```python
from build123d import *
from OCP.BRepFilletAPI import BRepFilletAPI_MakeChamfer

# Parameters (mm, degrees)
SKETCH1_R            = 4.999999999999999
SKETCH1_R_2          = 2.5
BOSS_EXTRUDE1_DEPTH  = 15.8
SKETCH2_R            = 3.75
CUT_EXTRUDE1_DEPTH   = 13
CUT_EXTRUDE2_DEPTH   = 19.135324645563973
BOSS_EXTRUDE3_DEPTH  = 1
BOSS_EXTRUDE4_DEPTH  = 1
SKETCH13_R           = 5
BOSS_EXTRUDE7_DEPTH  = 10
CUT_EXTRUDE3_START   = -4
CUT_EXTRUDE3_DEPTH   = 4
CUT_EXTRUDE4_DEPTH   = 1
BOSS_EXTRUDE9_DEPTH  = 3
CUT_EXTRUDE6_DEPTH   = 7
BOSS_EXTRUDE10_DEPTH = 3
BOSS_EXTRUDE11_DEPTH = 2
CUT_EXTRUDE7_DEPTH   = 0.25
BOSS_EXTRUDE12_DEPTH = 1
SKETCH23_W           = 18.9749371855331
SKETCH23_H           = 13
BOSS_EXTRUDE13_DEPTH = 1
SKETCH24_W           = 23.799999999999997
SKETCH24_H           = 13
BOSS_EXTRUDE14_DEPTH = 1
BOSS_EXTRUDE15_DEPTH = 1
SKETCH26_W           = 11.45
SKETCH26_H           = 6.999999999999998
SKETCH26_W_2         = 10.45
SKETCH26_H_2         = 5.999999999999998
CUT_EXTRUDE8_DEPTH   = 34.46489573009899
CUT_EXTRUDE10_DEPTH  = 0.7
CHAMFER4_SIZE        = 0.8
CHAMFER4_SIZE2       = 2.1979819355637176


with BuildPart() as part:
    # Sketch1 → Boss-Extrude1 (new body)
    # profile 1 of 2: a face of its own
    with BuildSketch(Plane(origin=(0, 0, 0), x_dir=(1, 0, 0), z_dir=(0, 1, 0))):
        with BuildLine():
            Line((-0.5, 7), (-0.5, 4.9749371855331))
            ThreePointArc((-0.5000000000000004, 4.974937185533099), (3.1e-16, 4.999999999999999), (0.49999999999999994, 4.974937185533099))
            Line((0.5, 4.9749371855331), (0.5, 7))
            Line((0.5, 7), (-0.5, 7))
        make_face()
    # profile 2 of 2: a face of its own
    with BuildSketch(Plane(origin=(0, 0, 0), x_dir=(1, 0, 0), z_dir=(0, 1, 0))):
        Circle(SKETCH1_R)
        with Locations(Location((0, 0, 0), (0, 0, 270))):
            Circle(SKETCH1_R_2, mode=Mode.SUBTRACT)
    extrude(amount=BOSS_EXTRUDE1_DEPTH)

    # Sketch2 → Cut-Extrude1 (cut)
    with BuildSketch(Plane(origin=(0, 15.8, 0), x_dir=(1, 0, 0), z_dir=(0, 1, 0))):
        with Locations(Location((0, 0, 0), (0, 0, 270))):
            Circle(SKETCH2_R)
    extrude(amount=-CUT_EXTRUDE1_DEPTH, mode=Mode.SUBTRACT)

    # Sketch4 → Cut-Extrude2 (cut, through all)
    with BuildSketch(Plane(origin=(0.5, 0, 0), x_dir=(0, 0, -1), z_dir=(1, 0, 0))):
        Polygon((7, 0), (4.9749371855331, 0), (4.9749371855331, 2.5000000000000004), (7, 2.5), align=None)
    extrude(amount=-CUT_EXTRUDE2_DEPTH, mode=Mode.SUBTRACT)

    # Sketch10 → Boss-Extrude3 (add)
    with BuildSketch(Plane(origin=(0.5, 0, 0), x_dir=(0, 0, -1), z_dir=(1, 0, 0))):
        Polygon((4.9749371855331, 15.8), (9.974937185533099, 15.8), (9.974937185533099, 9.8), (4.974937185533101, 9.8), align=None)
    extrude(amount=-BOSS_EXTRUDE3_DEPTH)

    # Sketch12 → Boss-Extrude4 (add)
    with BuildSketch(Plane(origin=(0, 15.8, 0), x_dir=(1, 0, 0), z_dir=(0, 1, 0))):
        with BuildLine():
            Line((-3.75, -3.307189138830739), (-3.75, 3.307189138830739))
            ThreePointArc((-3.75, 3.307189138830739), (-5.000000000000001, -6.1e-16), (-3.75, -3.307189138830739))
        make_face()
    extrude(amount=BOSS_EXTRUDE4_DEPTH)

    # Sketch13 → Boss-Extrude7 (add)
    with BuildSketch(Plane.XZ.offset(-9.8)):
        Polygon((-8, 8), (14.799999999999997, 8), (14.8, -9.974937185533099), (-7.999999999999998, -9.974937185533099), align=None)
        with Locations(Location((0, 0, 0), (0, 0, 221.409622109))):
            Circle(SKETCH13_R, mode=Mode.SUBTRACT)
    extrude(amount=-BOSS_EXTRUDE7_DEPTH)

    # Sketch14 → Cut-Extrude3 (cut)
    with BuildSketch(Plane(origin=(0, 19.8, 0), x_dir=(1, 0, 0), z_dir=(0, 1, 0)).offset(CUT_EXTRUDE3_START)):
        Polygon((-4.400000000000001, 5.7), (10.299999999999999, 5.7), (12.899999999999999, 5.7), (12.899999999999999, -7.249999999999999), (10.3, -7.249999999999999), (-4.400000000000001, -7.249999999999999), align=None)
    extrude(amount=CUT_EXTRUDE3_DEPTH, mode=Mode.SUBTRACT)

    # Sketch15 → Cut-Extrude4 (cut)
    with BuildSketch(Plane(origin=(0, 19.8, 0), x_dir=(1, 0, 0), z_dir=(0, 1, 0))):
        Polygon((-7.499999999999998, 9.474937185533099), (-7.5, -7.5), (14.299999999999997, -7.5), (14.3, 9.474937185533099), align=None)
    extrude(amount=-CUT_EXTRUDE4_DEPTH, mode=Mode.SUBTRACT)

    # Sketch17 → Boss-Extrude9 (add)
    with BuildSketch(Plane.XZ.offset(-9.8)):
        Polygon((14.8, -5.974937185533098), (4.3, -5.974937185533099), (4.3, 8), (14.8, 8), align=None)
    extrude(amount=BOSS_EXTRUDE9_DEPTH)

    # Sketch16 → Cut-Extrude6 (cut)
    with BuildSketch(Plane(origin=(0, 15.8, 0), x_dir=(1, 0, 0), z_dir=(0, 1, 0))):
        Polygon((12.899999999999999, 5.7), (4.999999999999999, 5.699999999999999), (5.000000000000001, -7.249999999999999), (12.9, -7.249999999999999), align=None)
    extrude(amount=-CUT_EXTRUDE6_DEPTH, mode=Mode.SUBTRACT)

    # Sketch19 → Boss-Extrude10 (add)
    with BuildSketch(Plane(origin=(0, 19.8, 0), x_dir=(1, 0, 0), z_dir=(0, 1, 0))):
        Polygon((-7.999999999999998, 9.974937185533099), (-8, -8), (14.799999999999997, -8), (14.8, 9.974937185533099), align=None)
        Polygon((-7.5, -7.5), (14.299999999999997, -7.5), (14.3, 9.474937185533099), (-7.499999999999998, 9.474937185533099), align=None, mode=Mode.SUBTRACT)
    extrude(amount=BOSS_EXTRUDE10_DEPTH)

    # Sketch20 → Boss-Extrude11 (add)
    with BuildSketch(Plane(origin=(0, 16.8, 0), x_dir=(1, 0, 0), z_dir=(0, 1, 0))):
        with BuildLine():
            Line((-4.400000000000002, -2.37486841740758), (-4.400000000000001, 2.374868417407581))
            ThreePointArc((-4.400000000000001, 2.374868417407581), (-5, 6.1e-16), (-4.400000000000002, -2.37486841740758))
        make_face()
    extrude(amount=BOSS_EXTRUDE11_DEPTH)

    # Sketch21 → Cut-Extrude7 (cut)
    with BuildSketch(Plane(origin=(0, 0, 7.249999999999999), x_dir=(-1, 0, 0), z_dir=(0, 0, -1))):
        Polygon((4.400000000000001, 18.8), (-12.899999999999999, 18.8), (-12.9, 8.800000000000002), (-5.000000000000001, 8.800000000000002), (-5.000000000000001, 15.8), (4.400000000000001, 15.8), align=None)
    extrude(amount=-CUT_EXTRUDE7_DEPTH, mode=Mode.SUBTRACT)

    # Sketch22 → Boss-Extrude12 (add)
    with BuildSketch(Plane.XY.offset(8)):
        Polygon((14.8, 6.800000000000002), (14.799999999999997, 22.8), (-8, 22.8), (-8, 9.8), (4.3, 9.8), (4.3, 6.800000000000002), align=None)
    extrude(amount=BOSS_EXTRUDE12_DEPTH)

    # Sketch23 → Boss-Extrude13 (add)
    with BuildSketch(Plane.ZY.offset(8)):
        with Locations((-0.4874685927665485, 16.3)):
            Rectangle(SKETCH23_W, SKETCH23_H)
    extrude(amount=BOSS_EXTRUDE13_DEPTH)

    # Sketch24 → Boss-Extrude14 (add)
    with BuildSketch(Plane(origin=(0, 0, -9.974937185533099), x_dir=(-1, 0, 0), z_dir=(0, 0, -1))):
        with Locations((-2.9000000000000012, 16.3)):
            Rectangle(SKETCH24_W, SKETCH24_H)
    extrude(amount=BOSS_EXTRUDE14_DEPTH)

    # Sketch25 → Boss-Extrude15 (add)
    with BuildSketch(Plane(origin=(14.799999999999999, 0, 2.86e-15), x_dir=(1.9e-16, 0, -1), z_dir=(1, 0, 1.9e-16))):
        Polygon((5.974937185533101, 9.8), (10.974937185533104, 9.8), (10.974937185533104, 22.8), (-8.999999999999998, 22.8), (-8.999999999999998, 6.800000000000002), (5.974937185533101, 6.800000000000002), align=None)
    extrude(amount=BOSS_EXTRUDE15_DEPTH)

    # Sketch26 → Cut-Extrude8 (cut, through all)
    with BuildSketch(Plane.ZY.offset(-12.899999999999999)):
        with Locations((0.42500000000000027, 12.8)):
            Rectangle(SKETCH26_W, SKETCH26_H)
        with Locations((0.4249999999999998, 12.8)):
            Rectangle(SKETCH26_W_2, SKETCH26_H_2)
    extrude(amount=-CUT_EXTRUDE8_DEPTH, mode=Mode.SUBTRACT)

    # Sketch28 → Cut-Extrude10 (cut)
    with BuildSketch(Plane.XZ.offset(-6.800000000000002)):
        with BuildLine():
            Line((4.3, -2.551470164434614), (4.3, -5.974937185533099))
            Line((4.3, -5.974937185533099), (15.8, -5.974937185533098))
            Line((15.8, -5.974937185533098), (15.799999999999999, 9.000000000000002))
            Line((15.799999999999999, 9.000000000000002), (4.3, 9.000000000000002))
            Line((4.3, 9.000000000000002), (4.3, 2.5514701644346127))
            ThreePointArc((4.3, 2.5514701644346127), (4.999999999999999, -5.6e-16), (4.3, -2.551470164434614))
        make_face()
    extrude(amount=-CUT_EXTRUDE10_DEPTH, mode=Mode.SUBTRACT)

    # Chamfer4: one chamfer whose edges measure the first distance from different faces: ONE call of the kernel's chamfer builder (chamfer() names one face for all edges)
    chamfer4_edges_1 = [part.edges().sort_by_distance(p)[0] for p in [
        (10.05, 7.500000000000002, -5.974937185533099),
    ]]
    chamfer4_side_1 = [part.faces().sort_by_distance(p)[0] for p in [
        (10.049999999999999, 8.65, -5.974937185533099),
    ]]
    chamfer4_edges_2 = [part.edges().sort_by_distance(p)[0] for p in [
        (4.3, 7.500000000000002, -4.263203674983856),
    ]]
    chamfer4_side_2 = [part.faces().sort_by_distance(p)[0] for p in [
        (4.3, 8.650000000000002, -4.263203674983856),
    ]]
    chamfer4 = BRepFilletAPI_MakeChamfer(part.part.solid().wrapped)
    for e in chamfer4_edges_1:
        chamfer4.Add(CHAMFER4_SIZE, CHAMFER4_SIZE2, e.wrapped, chamfer4_side_1[0].wrapped)  # the first distance lies on this face
    for e in chamfer4_edges_2:
        chamfer4.Add(CHAMFER4_SIZE, CHAMFER4_SIZE2, e.wrapped, chamfer4_side_2[0].wrapped)  # the first distance lies on this face
    add(Compound.cast(chamfer4.Shape()), mode=Mode.REPLACE)


solid = part.part
```
Design review of the part built by this model. Coordinates are the model's own, in mm. A direction names the side the tool comes from. Give positions to 0.01 mm unless a question says otherwise; leave off trailing zeros. Write each loop counter-clockwise with the first axis right and the second up, starting at its lowest first coordinate (ties: lowest second). Pieces come first, ordered by that corner, then holes. Notation, with made-up numbers: (-13.5, 64) - (-7.5, 64) arc R27 cw to (-7.5, 101) - close; hole circle Ø6 at (-37, 82.25). An arc over 180 degrees is marked (long way). Return JSON: item names as keys, results as strings. Group by question number.
(1) We need section C-C, the plane y = 4.75. Give the boundary of the cut face in (x, z).
(2) We need section D-D, the plane x = 8.5. Give the boundary of the cut face in (y, z), then the cut area to 3 significant figures.
(3) To check wall thickness, follow probe 1 along X at (y, z) = (8.25, 0); probe 2 along Z at (x, y) = (0, 0.95); probe 3 along X at (y, z) = (10.75, 6.75). State the ranges of each line that lie inside material, in increasing order.
(4) Insertion check: pin 1 (6 mm diameter, centred on y = 10, z = 3.5, fed in from +X); pin 2 (4.5 mm diameter, centred on x = 0.5, z = -1, fed in from +Y); pin 3 (2.5 mm diameter, centred on x = 9, z = 3.5, fed in from +Y); pin 4 (2 mm diameter, centred on y = 6, z = -2.5, fed in from +X). Each pin has a flat end and moves straight along its axis. Give the tip position at first contact, or say it passes through.
(5) Machinability: for faces 5 (the flat face through (0.5, 6, -6)), 6 (the flat face through (4.3, 9, 6)), 7 (the flat face through (0, 2.5, -6)), 8 (the flat face through (6, 17, 7.5)), 9 (the flat face through (9.97, 7.894, -4.861)), which of the approach directions +Z, -Z, +X, -X, +Y, -Y give a long, thin tool a straight path to every point of the face, cutting with its end or side? Answer none if there is none.
(6) Mouldability with a two-part tool opening along Y and no side actions: class faces 1 (the flat face through (14, 13, -5.3)), 2 (the cylindrical face through (-2.44, 1.38, -0.54)), 3 (the flat face through (5.4, 7.9, 1.6)), 4 (the flat face through (3, 2.8, 0)) as +Y half, -Y half, draft (parallel to the pull), parting line (faces both ways), or undercut.
(7) We need section A-A, the plane x = 0. Give the boundary of the cut face in (y, z).
(8) We need section B-B, the plane z = 0. Give the number of separate pieces and of enclosed holes in the cut face, then the cut area to 3 significant figures.
Reported:
{
 "1": {"outline": "(-0.5, -7) - (0.5, -7) - (0.5, -4.97) arc R5 ccw (long way) to (-0.5, -4.97) - close; hole circle Ø7.5 at (0, 0)"},
 "2": {"outline": "(7.5, -3.78) - (8.3, -5.97) - (9.8, -5.97) - (9.8, -10.97) - (22.8, -10.97) - (22.8, -9.47) - (18.8, -9.47) - (18.8, -5.7) - (8.8, -5.7) - (8.8, 7.5) - (22.8, 7.5) - (22.8, 9) - (7.5, 9) - close", "area": "93.3 mm2"},
 "3": {"probe 1": "x = -5 to -3.75, 3.75 to 15.8", "probe 2": "z = -4.97 to -2.5, 2.5 to 5", "probe 3": "x = -9 to 5, 12.9 to 15.8"},
 "4": {"pin 1": "stops at x = 15.8", "pin 2": "stops at y = 2.8", "pin 3": "stops at y = 8.8", "pin 4": "stops at x = 4.77"},
 "5": {"face 5": "-Z, -Y", "face 6": "+Z, -Y", "face 7": "-Z, +X, -X, -Y", "face 8": "+Y", "face 9": "-Z, +X, -Y"},
 "6": {"face 1": "undercut", "face 2": "draft", "face 3": "-Y half", "face 4": "+Y half"},
 "7": {"outline": "(0, -4.97) - (2.5, -4.97) - (2.5, -7) - (9.8, -7) - (9.8, -10.97) - (22.8, -10.97) - (22.8, -9.47) - (18.8, -9.47) - (18.8, -5.7) - (15.8, -5.7) - (15.8, -3.75) - (2.8, -3.75) - (2.8, -2.5) - (0, -2.5) - close; (0, 2.5) - (2.8, 2.5) - (2.8, 3.75) - (15.8, 3.75) - (15.8, 7.5) - (22.8, 7.5) - (22.8, 9) - (9.8, 9) - (9.8, 5) - (0, 5) - close"},
 "8": {"separate pieces": "3", "enclosed holes": "0", "area": "119 mm2"}
}
